from build123d import *

# Parameters (mm, degrees)
F0_R          = 3.175
F1_DEPTH      = 3.81
F1_DEPTH_BACK = 3.81
F2_R          = 3.175
F3_DEPTH      = 3.4925
F3_DEPTH_BACK = 11.1125
F5_R          = 5.08
F6_R          = 7.62
F8_DEPTH      = 7.3025
F8_DEPTH_BACK = 7.3025
F4_W          = 35.6460946558
F4_H          = 8.89
F4_W_2        = 48.26
F4_W_3        = 30.9916705634
F9_DEPTH      = 23.5553863263
F10_T1_DEPTH  = 7.62
F10_T3_DEPTH  = 40.2569110938
F10_T5_DEPTH  = 13.2510444311
F10_T7_DEPTH  = 40.2569110938


# Not quite as in the source:
# - a fillet or chamfer that OpenCascade refuses, or shapes differently, is made with other operations: its cross-section is extruded or revolved along the edge and cut away or added


with BuildPart() as f1:
    # F0 (on Top) → F1 (new body, two sides)
    with BuildSketch(Plane.XY) as f1_sk:
        with BuildLine():
            Line((17.1451295545, 8.0645), (21.8027879538, 8.0645))
            ThreePointArc((21.8027879538, 8.0645), (28.7489728397, 4.0971545957), (28.860781215, -3.9013960801))
            Line((28.860781215, -3.9013960801), (42.9672120462, 20.531658833))
            Line((42.9672120462, 20.531658833), (102.5673909916, 62.2641534092))
            Line((102.5673909916, 62.2641534092), (93.2803106107, 75.5274787436))
            Line((93.2803106107, 75.5274787436), (30.8609248359, 31.8209542937))
            Line((30.8609248359, 31.8209542937), (17.1451295545, 8.0645))
        make_face()
        with BuildLine():
            ThreePointArc((28.7104927, -4.1617034239), (28.7868498226, -4.03225), (28.860781215, -3.9013960801))
            Line((28.860781215, -3.9013960801), (28.7104927, -4.1617034239))
        make_face()
        with BuildLine():
            ThreePointArc((28.860781215, -3.9013960801), (28.7489728397, 4.0971545957), (21.8027879538, 8.0645))
            Line((21.8027879538, 8.0645), (17.1451295545, 8.0645))
            Line((17.1451295545, 8.0645), (-21.8027879538, 8.0645))
            ThreePointArc((-21.8027879538, 8.0645), (-29.8672879538, 0), (-21.8027879538, -8.0645))
            Line((-21.8027879538, -8.0645), (21.8027879538, -8.0645))
            Line((21.8027879538, -8.0645), (26.4572120462, -8.0645))
            Line((26.4572120462, -8.0645), (28.7104927, -4.1617034239))
            Line((28.7104927, -4.1617034239), (28.860781215, -3.9013960801))
        make_face()
        with Locations((-21.8027879538, 0)):
            Circle(F0_R, mode=Mode.SUBTRACT)
        with Locations((21.8027879538, 0)):
            Circle(F0_R, mode=Mode.SUBTRACT)
    extrude(amount=F1_DEPTH)
    extrude(f1_sk.sketch, amount=-F1_DEPTH_BACK)

    # F2 (on face) → F3 (join, two sides)
    with BuildSketch(Plane.XY.offset(3.81)) as f3_sk:
        with BuildLine():
            Line((17.1451295545, 8.0645), (-21.8027879538, 8.0645))
            ThreePointArc((-21.8027879538, 8.0645), (-29.8672879538, 0), (-21.8027879538, -8.0645))
            Line((-21.8027879538, -8.0645), (26.4572120462, -8.0645))
            Line((26.4572120462, -8.0645), (28.7104927, -4.1617034239))
            ThreePointArc((28.7104927, -4.1617034239), (28.7868498226, -4.03225), (28.860781215, -3.9013960801))
            ThreePointArc((28.860781215, -3.9013960801), (28.7489728397, 4.0971545957), (21.8027879538, 8.0645))
            Line((21.8027879538, 8.0645), (17.1451295545, 8.0645))
        make_face()
        with Locations((-21.8027879538, 0)):
            Circle(F2_R, mode=Mode.SUBTRACT)
        with Locations((21.8027879538, 0)):
            Circle(F2_R, mode=Mode.SUBTRACT)
    extrude(amount=F3_DEPTH)
    extrude(f3_sk.sketch, amount=-F3_DEPTH_BACK)

    # F5
    f5_edges = [f1.edges().sort_by_distance(p)[0] for p in [
        (26.457212, -8.0645, 0),
        (17.14513, 8.0645, 0),
    ]]
    fillet(f5_edges, radius=F5_R)

    # F6
    f6_edges = [f1.edges().sort_by_distance(p)[0] for p in [
        (93.280311, 75.527479, 0),
        (102.567391, 62.264153, 0),
    ]]
    fillet(f6_edges, radius=F6_R)

    # F7 (on Top) → F8 (join, two sides)
    with BuildSketch(Plane.XY) as f8_sk:
        with BuildLine():
            Line((26.088796945, 23.5553863263), (18.6115992382, 10.6045))
            ThreePointArc((18.6115992382, 10.6045), (16.752190187, 8.7450909488), (14.212190187, 8.0645))
            Line((14.212190187, 8.0645), (21.8027879538, 8.0645))
            ThreePointArc((21.8027879538, 8.0645), (28.7489728397, 4.0971545957), (28.860781215, -3.9013960801))
            Line((28.860781215, -3.9013960801), (40.0569206826, 15.4908863263))
            Line((40.0569206826, 15.4908863263), (26.088796945, 23.5553863263))
        make_face()
    extrude(amount=F8_DEPTH)
    extrude(f8_sk.sketch, amount=-F8_DEPTH_BACK)

    # F4 (on face) → F9 (cut, through all)
    with BuildSketch(Plane.XZ.offset(8.0645)):
        with Locations((-39.6258352817, 0)):
            Rectangle(F4_W, F4_H)
        with Locations((2.3272120462, 0)):
            Rectangle(F4_W_2, F4_H)
        with Locations((41.9530473279, 0)):
            Rectangle(F4_W_3, F4_H)
    extrude(amount=-F9_DEPTH, mode=Mode.SUBTRACT)

    # F10: fillet of radius 5.08 on 4 edges, made by hand

    # F10_s2 → F10_t1 (join)
    with BuildSketch(Plane.XY.offset(-3.81)):
        with BuildLine():
            ThreePointArc((43.8897483577, 21.1776257125), (43.0581477833, 20.4483315822), (42.4041076031, 19.5563333275))
            Line((42.4041076031, 19.5563333275), (42.9672120462, 20.531658833))
            Line((42.9672120462, 20.531658833), (43.8897483577, 21.1776257125))
        make_face()
    extrude(amount=F10_T1_DEPTH)

    # F10_s4 → F10_t3 (cut)
    with BuildSketch(Plane(origin=(33.7826319428, -19.5044116461, 0), x_dir=(0, 0, 1), z_dir=(-0.8660254038, 0.5, 0))):
        with BuildLine():
            ThreePointArc((-3.81, 33.4439614271), (-6.3377703435, 31.5967932158), (-7.3025, 28.6183792083))
            Line((-7.3025, 28.6183792083), (-7.3025, 33.4439614271))
            Line((-7.3025, 33.4439614271), (-3.81, 33.4439614271))
        make_face()
    extrude(amount=F10_T3_DEPTH, mode=Mode.SUBTRACT)

    # F10_s6 → F10_t5 (cut)
    with BuildSketch(Plane.XY.offset(-6.6255222156)):
        with BuildLine():
            ThreePointArc((31.7834611474, 32.4669211732), (30.951860573, 31.7376270429), (30.2978203928, 30.8456287882))
            Line((30.2978203928, 30.8456287882), (30.8609248359, 31.8209542937))
            Line((30.8609248359, 31.8209542937), (31.7834611474, 32.4669211732))
        make_face()
    extrude(amount=F10_T5_DEPTH, mode=Mode.SUBTRACT)

    # F10_s8 → F10_t7 (cut)
    with BuildSketch(Plane(origin=(33.7826319428, -19.5044116461, 0), x_dir=(0, 0, 1), z_dir=(-0.8660254038, 0.5, 0))):
        with BuildLine():
            ThreePointArc((7.3025, 28.6183792083), (6.3377703435, 31.5967932158), (3.81, 33.4439614271))
            Line((3.81, 33.4439614271), (7.3025, 33.4439614271))
            Line((7.3025, 33.4439614271), (7.3025, 28.6183792083))
        make_face()
    extrude(amount=F10_T7_DEPTH, mode=Mode.SUBTRACT)


solid = f1.part
Build history of the part. All positions in model axes, mm. A direction names the side the tool comes from. Give positions to 0.01 mm unless a question says otherwise; leave off trailing zeros. Write each loop counter-clockwise with the first axis right and the second up, starting at its lowest first coordinate (ties: lowest second). Pieces come first, ordered by that corner, then holes. Notation, with made-up numbers: (-39, 32) - (6, 32) arc R13 ccw to (6, 43) - close; hole circle Ø7 at (12, -35). An arc over 180 degrees is marked (long way). Use one line per item in the form item = value. Start each with the question number.
1. Probe line 1 (Z direction, x = -14, y = 3.5) (1 decimal); line 2 (X direction, y = 0, z = 6.25); line 3 (Y direction, x = 9.5, z = 6.25). List the from-to ranges inside material, lowest first. Write a range as [from, to].
2. Band-saw the part on C-C on y = 66.5. Write the cut outline in (x, z), plus the area to 3 significant figures.
3. 3-axis set-ups, long thin cutter, end or side, ignore diameter. For faces 5 (the face through (99.473, 62.895, 0.053)), 6 (the face through (-4, 8.065, -6)), 7 (the face through (5, 1, -4.445)): which of +Z, -Z, +X, -X, +Y, -Y reach the whole face in a straight line?
4. Band-saw the part on B-B on z = 1.5. Write the cut outline in (x, y), plus the area to 3 significant figures.
5. Drop flat-ended pins along their axis: pin 1 Ø1.4 at (x, z) = (-1.5, -5.5) entering from +Y; pin 2 Ø3 at (x, z) = (82, 0) entering from +Y; pin 3 Ø4 at (y, z) = (43, -3.5) entering from -X. Give the stop position or say it passes through.
6. Two-plate mould, pull along X, no slides. Class faces 1 (the face through (16.78, 8.76, 5.89)), 2 (the face through (24.831, 0.954, 5.854)), 3 (the face through (92.65, 72.433, 0.053)), 4 (the face through (32.27, 17.9, -6.31)): released by +X, released by -X, zero draft, split by the parting line, or undercut.
7. Band-saw the part on D-D on y = 47. Write the cut outline in (x, z), plus the area to 3 significant figures.
8. Band-saw the part on A-A on y = 0. Write the cut outline in (x, z) (1 decimal), plus the area to 3 significant figures.
Conclusion:
q1.line_1 = [-7.3, -4.4], [4.4, 7.3]
q1.line_2 = [-29.87, -24.98], [-18.63, 18.63], [24.98, 31.11]
q1.line_3 = [-8.06, 8.06]
q2.outline = (80.39, -3.81) - (99.2, -3.81) - (99.2, 3.81) - (80.39, 3.81) - close
q2.area = 143 mm²
q3.face_5 = +Z, -Z, +X
q3.face_6 = +Z, -Z, -X, +Y
q3.face_7 = +X, -X, -Y
q4.outline = (21.43, 15.49) - (40.06, 15.49) - (42.4, 19.56) arc R5.08 cw to (43.89, 21.18) - (96.33, 57.89) arc R7.62 ccw to (98.2, 68.51) - (97.65, 69.29) arc R7.62 ccw to (87.04, 71.16) - (31.78, 32.47) arc R5.08 ccw to (30.3, 30.85) - close
q4.area = 1,380 mm²
q5.pin_1 = 8.06
q5.pin_2 = 68.68
q5.pin_3 = 43.97
q6.face_1 = released by -X
q6.face_2 = undercut
q6.face_3 = split by the parting line
q6.face_4 = released by +X
q7.outline = (52.54, -3.81) - (80.77, -3.81) - (80.77, 3.81) - (52.54, 3.81) - close
q7.area = 215 mm²
q8.outline = (-29.9, -7.3) - (-25, -7.3) - (-25, -4.4) - (-29.9, -4.4) - close; (-29.9, 4.4) - (-25, 4.4) - (-25, 7.3) - (-29.9, 7.3) - close; (-18.6, -7.3) - (18.6, -7.3) - (18.6, -4.4) - (-18.6, -4.4) - close; (-18.6, 4.4) - (18.6, 4.4) - (18.6, 7.3) - (-18.6, 7.3) - close; (25, -7.3) - (31.1, -7.3) - (31.1, -4.4) - (25, -4.4) - close; (25, 4.4) - (31.1, 4.4) - (31.1, 7.3) - (25, 7.3) - close
q8.area = 276 mm²
